For this review, take the finished solid that the model builds, in its own axes (mm). Face numbers are marked on the shaded views. A direction names the side the tool comes from. Round coordinates to 2 decimals unless told otherwise and drop trailing zeros. Order: outer loops, then holes, each group sorted by start corner. A loop starts at its lowest first (then second) coordinate and runs counter-clockwise, first axis right, second up. Notation, with made-up numbers: (24, -31) -> (83, -31) arc R25 ccw to (83, -11) -> close; hole circle Ø2 at (-2, 82). An arc over 180 degrees is marked (long way). Put each result on its own line as item: value. Start each with the question number.
Autodesk Inventor part; units mm, degrees
ref_plane "YZ Plane" through (0, 0, 0) normal (1, 0, 0) x (0, 1, 0)
ref_plane "XZ Plane" through (0, 0, 0) normal (0, 1, 0) x (-1, 0, 0)
ref_plane "XY Plane" through (0, 0, 0) normal (0, 0, 1) x (1, 0, 0)
sketch "Sketch1" plane through (0, 0, 0) normal (0, 0, 1) x (1, 0, 0)
  line L0 (6, 0) -> (6, 2)
  line L1 (6, 0) -> (1, 0)
  line L2 (6, 2) -> (-6, 2)
  line L3 (-6, 2) -> (-6, 0)
  line L4 (-6, 0) -> (-1, 0)
  line L5 (-8, -8) -> (-7, -6)
  line L6 (8, -8) -> (7, -6)
  line L7 (-7, -6) -> (-2, -6)
  line L8 (-1, 0) -> (-1, -5)
  arc A0 (-2, -6) -> (-1, -5) centre (-2, -5) ccw
  line L9 (-8, -8) -> (-2, -8)
  line L10 (-2, -8) -> (-1, -7)
  line L11 (-1, -7) -> (1, -7)
  line L12 (1, -7) -> (2, -8)
  line L13 (2, -8) -> (8, -8)
  line L14 (1, 0) -> (1, -5)
  line L15 (7, -6) -> (2, -6)
  arc A1 (1, -5) -> (2, -6) centre (2, -5) ccw
  point P0 (0, 0)
  dimension "d0" = 6
  dimension "d1" = 2
  dimension "d3" = 5
  dimension "d6" = 12
  dimension "d7" = 2
  dimension "d8" = 5
  dimension "d26" = 5
  dimension "d27" = 5
  dimension "d28" = 6
  dimension "d29" = 5
  dimension "d30" = 5
  dimension "d49" = 2
  dimension "d50" = 2
  dimension "d51" = 1
revolve "Revolution1" add sketch "Sketch1" angle 360 about axis through (6, 2, 0) along (-1, 0, 0)
sketch "Sketch2" plane through (1, 2, 0) normal (1, 0, 0) x (0, 0, -1)
  circle A0 centre (0, 0) radius 8
  line L0 (0, 8) -> (0, 5)
  line L1 (-8, 0) -> (-5, 0)
  line L2 (0, -8) -> (0, -5)
  line L3 (8, 0) -> (5, 0)
  point P0 (0, -2)
  dimension "d15" = 3
  dimension "d16" = 3
  dimension "d17" = 3
  dimension "d18" = 3
hole "Hole1" [suppressed]
sketch "Sketch3" plane through (1, 2, 0) normal (1, 0, 0) x (0, 0, -1)
  line L0 (0, 2.0456) -> (0, 5.0456)
  circle A0 centre (0, 0) radius 2
  line L1 (-2, 0) -> (-5, 0)
  line L2 (0, -2) -> (0, -5)
  line L3 (2, 0) -> (5, 0)
  dimension "d31" = 3
  dimension "d32" = 3
  dimension "d33" = 3
  dimension "d34" = 3
hole "Hole2" at (1, 7.0456, 0) at (1, 2, -5) at (1, -3, 0) at (1, 2, 5) direction (-1, 0, 0) diameter 4 depth 8
sketch "Sketch5" plane through (6, 2, 0) normal (1, 0, 0) x (0, 0, -1)
  point P0 (0, 0)
  point P1 (0, 0)
hole "Hole3" at (6, 2, 0) direction (-1, 0, 0) diameter 2 depth 20
properties part number "Tank Wheel"
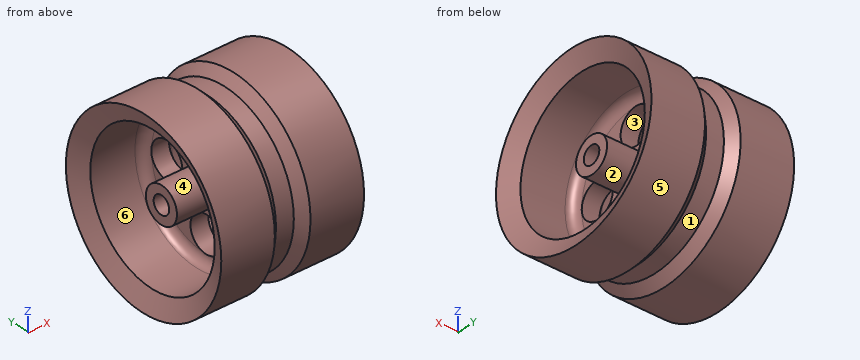
Item 1: Mouldability with a two-part tool opening along Y and no side actions: class the marked faces 5 and 6 as +Y half, -Y half, draft (parallel to the pull), parting line (faces both ways), or undercut.
Item 2: Insertion check: pin 1 Ø2 at (x, y) = (-3.5, 4.5) entering from -Z; pin 2 Ø5 at (y, z) = (-3, 0) entering from -X; pin 3 Ø1 at (x, z) = (4.5, -6) entering from -Y; pin 4 Ø3 at (y, z) = (2, -5) entering from +X. Each pin has a flat end and moves straight along its axis. Give the tip position at first contact, or say it passes through.
Item 3: Tool access review of the marked faces 1, 2, 3 and 4: name each direction out of +Z, -Z, +X, -X, +Y, -Y from which nothing blocks a thin tool from reaching the whole face with its end or side.
Item 4: For L1, parallel to Z at x = 3.55, y = 2; L2, parallel to Z at x = -0.1, y = 2; L3, parallel to Z at x = 1.5, y = 3.5, list the stretches that pass through material, from the lowest coordinate up.
Item 5: Consider section A-A, the plane x = -4.25. Write out the cut boundary in (y, z).
Evaluation:
1. face 5: parting line
1. face 6: undercut
2. pin 1: stops at z = -9.89
2. pin 2: stops at x = -1.13
2. pin 3: stops at y = -6.35
2. pin 4: passes through
3. face 1: none
3. face 2: +X
3. face 3: +X, -X
3. face 4: -X
4. L1: z = -10 to -8, -2 to -1, 1 to 2, 8 to 10
4. L2: z = -9 to -7, -3 to -1, 1 to 3, 7 to 9
4. L3: z = -9.38 to -7.72, -1.32 to 1.32, 7.72 to 9.38
5. outline: circle Ø20 at (2, 0); circle Ø4 at (2, 0); hole circle Ø16 at (2, 0); hole circle Ø2 at (2, 0)
